```python
from build123d import *

# Parameters (mm, degrees)
SKETCH_1_R      = 10
EXTRUDE_1_DEPTH = 10
SKETCH_2_R      = 10
EXTRUDE_2_DEPTH = 10


with BuildPart() as part:
    # 스케치1 → 보스-돌출1 (new body)
    with BuildSketch(Plane.XY):
        with BuildLine():
            Line((0, 20), (103.959759811, 20))
            ThreePointArc((103.959759811, 20), (123.959759811, 0), (103.959759811, -20))
            Line((103.959759811, -20), (0, -20))
            ThreePointArc((0, -20), (-20, 0), (0, 20))
        make_face()
        Circle(SKETCH_1_R, mode=Mode.SUBTRACT)
    extrude(amount=EXTRUDE_1_DEPTH)

    # 스케치2 → 보스-돌출2 (add)
    with BuildSketch(Plane(origin=(0, 0, 0), x_dir=(-1, 0, 0), z_dir=(0, 0, -1))):
        with Locations(Location((-103.959759811, 0, 0), (0, 0, 180))):
            Circle(SKETCH_2_R)
    extrude(amount=EXTRUDE_2_DEPTH)


solid = part.part
```
Work out the finished part from the listing and answer in its coordinate system (mm). A direction names the side the tool comes from. Give positions to 0.01 mm unless a question says otherwise; leave off trailing zeros. Order: outer loops, then holes, each group sorted by start corner. A loop starts at its lowest first (then second) coordinate and runs counter-clockwise, first axis right, second up.
1. For faces 4 (the flat face through (53, -20, 5)), 5 (the cylindrical face through (113.197, 3.83, -4.93)), determine the directions among +Z, -Z, +X, -X, +Y, -Y from which every point of the face is accessible in a straight line to the end or side of a thin tool.
Result sheet:
face 4: +Z, -Z, +X, -X, -Y
face 5: -Z
2. Each of these flat-tipped pins is pushed along its axis until it touches: P1, Ø4, axis at y = -8, z = 8, coming from the -X side; P2, Ø10, axis at x = 53, z = -2, coming from the -Y side; P3, Ø4, axis at y = -15.5, z = 3.5, coming from the +X side; P4, Ø6, axis at y = 4.5, z = 4, coming from the +X side. Where does it stop, or does it pass through?
Result sheet:
P1: stops at x = -19.08
P2: stops at y = -20
P3: stops at x = 118.72
P4: stops at x = 123.9
3. Section A-A, the plane y = 0 is taken. Determine the outline of the cut face in (x, z).
Result sheet:
outline: (-20, 0) - (-10, 0) - (-10, 10) - (-20, 10) - close; (10, 0) - (93.96, 0) - (93.96, -10) - (113.96, -10) - (113.96, 0) - (123.96, 0) - (123.96, 10) - (10, 10) - close
4. Straight lines are drawn through the part: L1, parallel to Y at x = 0, z = 4.25; L2, parallel to Z at x = -12, y = 13; L3, parallel to Y at x = -4, z = 2.75. For each, find the intervals that lie inside material, in ascending order.
Result sheet:
L1: y = -20 to -10, 10 to 20
L2: z = 0 to 10
L3: y = -19.6 to -9.17, 9.17 to 19.6
5. Section B-B, the plane z = 5.5 is taken. Determine the outline of the cut face in (x, y), and give its area (3 significant figures).
Result sheet:
outline: (0, -20) - (103.96, -20) arc R20 ccw to (103.96, 20) - (0, 20) arc R20 ccw to start; hole circle Ø20 at (0, 0)
area: 5,100 mm2
6. The mould has two halves that part along X. Classify faces 1 (the cylindrical face through (-2.17, -9.76, 4.93)), 2 (the cylindrical face through (123.955, 0.44, 4.93)), 3 (the flat face through (51, 20, 5)): released by +X, released by -X, zero draft, split by the parting line, or undercut.
Result sheet:
face 1: undercut
face 2: released by +X
face 3: zero draft
7. Section D-D, the plane y = -6 is taken. Determine the outline of the cut face in (x, z), and give its area (3 significant figures).
Result sheet:
outline: (-19.08, 0) - (-8, 0) - (-8, 10) - (-19.08, 10) - close; (8, 0) - (95.96, 0) - (95.96, -10) - (111.96, -10) - (111.96, 0) - (123.04, 0) - (123.04, 10) - (8, 10) - close
area: 1,420 mm2
8. Section C-C, the plane x = 106 is taken. Determine the outline of the cut face in (y, z).
Result sheet:
outline: (-19.9, 0) - (-9.79, 0) - (-9.79, -10) - (9.79, -10) - (9.79, 0) - (19.9, 0) - (19.9, 10) - (-19.9, 10) - close
